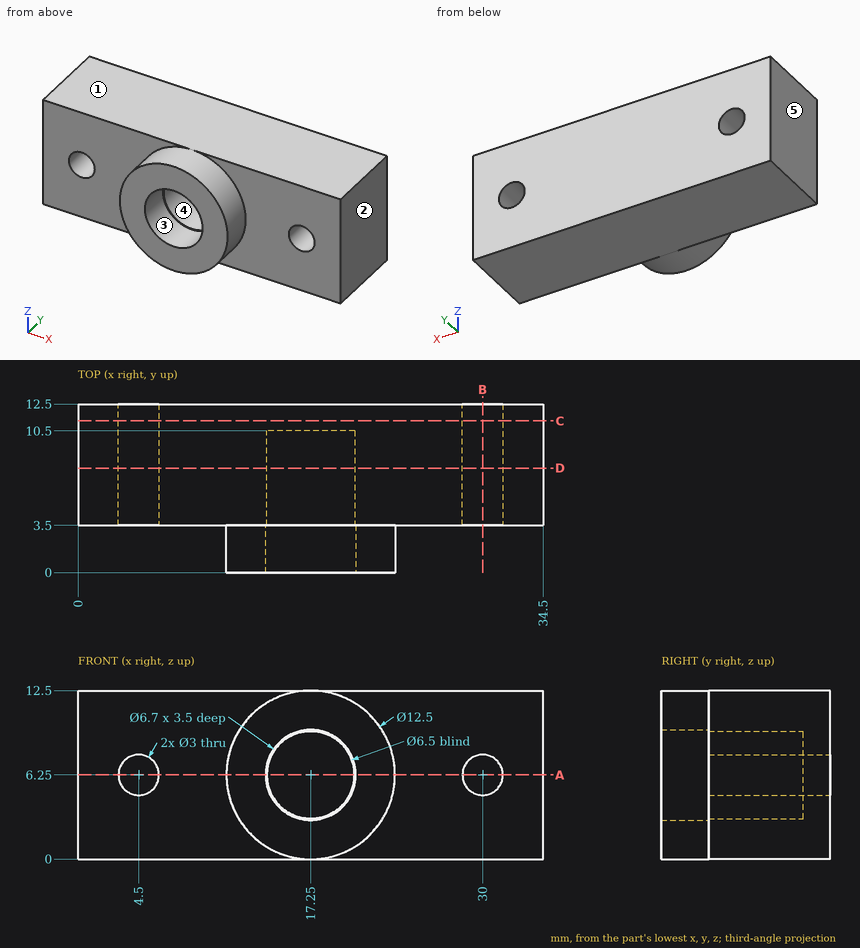
Verification items for this drawing (mm, ordinates from the low corner). A direction names the side the tool comes from. Give positions to 0.01 mm unless a question says otherwise; leave off trailing zeros. Write each loop counter-clockwise with the first axis right and the second up, starting at its lowest first coordinate (ties: lowest second). Pieces come first, ordered by that corner, then holes. Notation, with made-up numbers: (42, 71) - (81, 71) arc R27 cw to (81, 99) - close; hole circle Ø6 at (28, 75.5). An arc over 180 degrees is marked (long way). Answer as CSV lines item,"result". Start each with the question number.
1. Sectioned sample at B-B (x = 30). Record the boundary of the cut face in (y, z), then the cut area to 3 significant figures.
2. Sectioned sample at C-C (y = 11.25). Record the boundary of the cut face in (x, z), then the cut area to 3 significant figures.
3. Set-up check for the marked faces 4 and 5: record each of +Z, -Z, +X, -X, +Y, -Y from which the full face is reachable in a straight line by a thin tool's end or side.
4. Sectioned sample at D-D (y = 7.75). Record the boundary of the cut face in (x, z), then the cut area to 3 significant figures.
5. Depth check by flat-ended pin: pin 1 (1 mm diameter, centred on x = 5, z = 5, fed in from -Y); pin 2 (1 mm diameter, centred on x = 7.5, y = 2.5, fed in from +Z). Enter the tip coordinate at first touch or a pass-through.
6. Draft check along X on the marked faces 1, 2 and 3. Enter one of: pulls with the +X half, pulls with the -X half, needs draft (parallel to the pull), parting line crosses it, or undercut.
7. Sectioned sample at A-A (z = 6.25). Record the boundary of the cut face in (x, y), then the cut area to 3 significant figures.
8. Thickness scan on line 1 (Z direction, x = 17.25, y = 1.75); line 2 (Z direction, x = 30, y = 9.5); line 3 (Y direction, x = 7, z = 0.75). Record the ranges inside material, lowest first.
Derived:
1,outline,"(3.5, 0) - (12.5, 0) - (12.5, 4.75) - (3.5, 4.75) - close; (3.5, 7.75) - (12.5, 7.75) - (12.5, 12.5) - (3.5, 12.5) - close"
1,area,"85.5 mm²"
2,outline,"(0, 0) - (34.5, 0) - (34.5, 12.5) - (0, 12.5) - close; hole circle Ø3 at (4.5, 6.25); hole circle Ø3 at (30, 6.25)"
2,area,"417 mm²"
3,face 4,"-Y"
3,face 5,"+Z, -Z, -X, +Y, -Y"
4,outline,"(0, 0) - (34.5, 0) - (34.5, 12.5) - (0, 12.5) - close; hole circle Ø3 at (4.5, 6.25); hole circle Ø6.5 at (17.25, 6.25); hole circle Ø3 at (30, 6.25)"
4,area,"384 mm²"
5,pin 1,"y = 3.5"
5,pin 2,"through"
6,face 1,"needs draft"
6,face 2,"pulls with the +X half"
6,face 3,"undercut"
7,outline,"(0, 3.5) - (3, 3.5) - (3, 12.5) - (0, 12.5) - close; (6, 3.5) - (11, 3.5) - (11, 0) - (13.9, 0) - (13.9, 3.5) - (14, 3.5) - (14, 10.5) - (20.5, 10.5) - (20.5, 3.5) - (20.6, 3.5) - (20.6, 0) - (23.5, 0) - (23.5, 3.5) - (28.5, 3.5) - (28.5, 12.5) - (6, 12.5) - close; (31.5, 3.5) - (34.5, 3.5) - (34.5, 12.5) - (31.5, 12.5) - close"
7,area,"231 mm²"
8,line 1,"0 to 2.9, 9.6 to 12.5"
8,line 2,"0 to 4.75, 7.75 to 12.5"
8,line 3,"3.5 to 12.5"
